Here's how the part is built. I have some questions about the finished solid (model axes, mm). Face numbers are marked on the shaded views. A direction names the side the tool comes from. Round coordinates to 2 decimals unless told otherwise and drop trailing zeros. Write each loop counter-clockwise with the first axis right and the second up, starting at its lowest first coordinate (ties: lowest second). Pieces come first, ordered by that corner, then holes. Notation, with made-up numbers: (-26, 49) - (2, 49) arc R20 cw to (2, 86) - close; hole circle Ø5 at (48, 46.25). An arc over 180 degrees is marked (long way). Write item = value, one per line. Start each with the question number.
Item 1: Which directions (+Z, -Z, +X, -X, +Y, -Y) give clear straight access to the entire face, cutting with the end or side of a thin tool? Please do the marked faces 4 and 5.
Item 2: If we section it at B-B (z = 4.5): Give the number of separate pieces and of enclosed holes in the cut face, and give its area (3 significant figures).
Item 3: If we section it at D-D (x = 6): Please give me the cut outline in (y, z).
Item 4: For P1, Ø3.5, axis at x = 9, y = 0.5, coming from the +Z side; P2, Ø2, axis at y = -2, z = 5, coming from the +X side; P3, Ø2.5, axis at x = -9, y = 0.5, coming from the +Z side; P4, Ø1.5, axis at y = -2, z = 5, coming from the -X side, each with a flat end and sliding along its axis, tell me the tip position at first contact or that it passes through.
Item 5: If I drill on line 1 along Y through (x, z) = (-9, 1.75); line 2 along Y through (x, z) = (9, 4.95); line 3 along X through (y, z) = (0, 1.25), over which ranges is the centre line in solid material (lowest first)? Write a range as [from, to].
Item 6: If we section it at A-A (x = -9): Please give me the cut outline in (y, z), and give its area (3 significant figures).
Item 7: If we section it at C-C (y = 1.25): Please give me the cut outline in (x, z), and give its area (3 significant figures).
Item 8: Thinking about a two-plate mould opening in Y: for the marked faces 1, 2 and 3, which applies, pulls with the +Y half, pulls with the -Y half, needs draft (parallel to the pull), parting line crosses it, or undercut?
```python
from build123d import *

# Parameters (mm, degrees)
F0_W           = 20
F0_H           = 10
F1_DEPTH       = 6
F2_SIZE        = 9.99999
F3_R           = 4
F4_DEPTH       = 2.5
F6_D           = 3
F6_DEPTH       = 10
F6_CBORE_D     = 3
F6_CBORE_DEPTH = 10
F6_TIP         = 0.9012909285


# Not quite as in the source:
# - a fillet or chamfer is up to 0.001 mm smaller than in the source, because OpenCascade refuses the exact size


with BuildPart() as f1:
    # F0 (on Top) → F1 (new body)
    with BuildSketch(Plane.XY):
        with Locations((-10, 0)):
            Rectangle(F0_W, F0_H)
    extrude(amount=F1_DEPTH)

    # F2 (size 10 in the source; OpenCascade refuses exactly that, so slightly less here)
    f2_edges = [f1.edges().sort_by_distance(p)[0] for p in [
        (-20, -5, 3),
    ]]
    chamfer(f2_edges, length=F2_SIZE)

    # F3 (on face) → F4 (cut)
    with BuildSketch(Plane.XY.offset(6)):
        with Locations((-9, 0.5)):
            Circle(F3_R)
    extrude(amount=-F4_DEPTH, mode=Mode.SUBTRACT)

    # F6
    with Locations(Plane.XY.offset(3.5)):
        with Locations((-9, 0.5)):
            CounterBoreHole(F6_D / 2, F6_CBORE_D / 2, F6_CBORE_DEPTH, depth=F6_DEPTH)
            with Locations((0, 0, -(F6_DEPTH + F6_TIP / 2))):  # 118° drill point
                Cone(0, F6_D / 2, F6_TIP, mode=Mode.SUBTRACT)

    # F7: F1 across plane


with BuildPart() as f1_1:
    add(f1.part)
    add(f1.part.mirror(Plane.YZ))


solid = f1_1.part
```
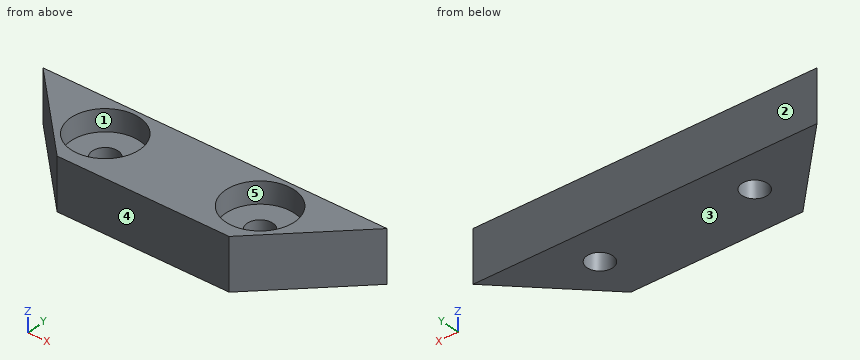
Reply:
q1.face_4 = +Z, -Z, +X, -X, -Y
q1.face_5 = +Z
q2.separate_pieces = 1
q2.enclosed_holes = 2
q2.area = 199 mm2
q3.outline = (-5, 0) - (5, 0) - (5, 6) - (3.15, 6) - (3.15, 3.5) - (-2.15, 3.5) - (-2.15, 6) - (-5, 6) - close
q4.P1 = 3.5
q4.P2 = 14
q4.P3 = through
q4.P4 = -13.75
q5.line_1 = [-5, -1], [2, 5]
q5.line_2 = [-5, -3.5], [4.5, 5]
q5.line_3 = [-15, -10.41], [-7.59, 7.59], [10.41, 15]
q6.outline = (-5, 0) - (-1, 0) - (-1, 3.5) - (-3.5, 3.5) - (-3.5, 6) - (-5, 6) - close; (2, 0) - (5, 0) - (5, 6) - (4.5, 6) - (4.5, 3.5) - (2, 3.5) - close
q6.area = 29.5 mm2
q7.outline = (-16.25, 0) - (-10.3, 0) - (-10.3, 3.5) - (-12.93, 3.5) - (-12.93, 6) - (-16.25, 6) - close; (-7.7, 0) - (7.7, 0) - (7.7, 3.5) - (5.07, 3.5) - (5.07, 6) - (-5.07, 6) - (-5.07, 3.5) - (-7.7, 3.5) - close; (10.3, 0) - (16.25, 0) - (16.25, 6) - (12.93, 6) - (12.93, 3.5) - (10.3, 3.5) - close
q7.area = 138 mm2
q8.face_1 = undercut
q8.face_2 = pulls with the +Y half
q8.face_3 = needs draft
